Drawing for the job (mm, zero at the part's lowest x, y, z). Give positions to 0.01 mm unless a question says otherwise; leave off trailing zeros. Write each loop counter-clockwise with the first axis right and the second up, starting at its lowest first coordinate (ties: lowest second). Pieces come first, ordered by that corner, then holes. Notation, with made-up numbers: M -3.5,19 L 44.5,19 A13 ccw 44.5,42 Z; hole C -22.75,14 d6. An arc over 180 degrees is marked long. Answer as a JSON object with one key per item and string values. Group by question number.
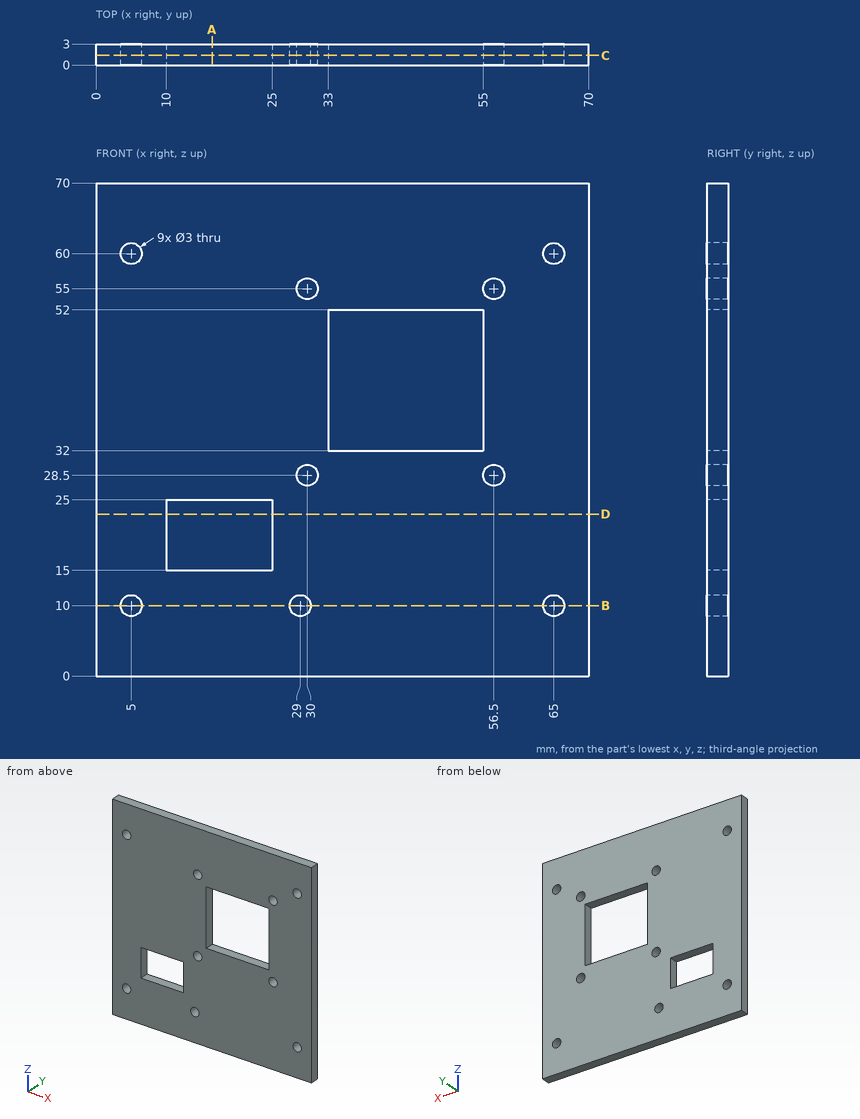
Q1. Slice it at C-C, the plane y = 1.4. Count the separate pieces of the cut face and the enclosed holes in it, then the cut area to 3 significant figures.
Q2. Wall check: L1, parallel to X at y = 1.55, z = 10; L2, parallel to X at y = 1.85, z = 60; L3, parallel to Z at x = 37.5, y = 2. Give the ranges that are in metal, low to high.
Q3. Slice it at A-A, the plane x = 16.5. Write the cut outline in (y, z), then the cut area to 3 significant figures.
Q4. Slice it at D-D, the plane z = 23. Write the cut outline in (x, y), then the cut area to 3 significant figures.
Q5. Drop flat-ended pins along their axis: P1, Ø4, axis at x = 30, z = 55, coming from the +Y side; P2, Ø2.5, axis at x = 65, z = 60, coming from the +Y side. Give the stop position or say it passes through.
Q6. Slice it at B-B, the plane z = 10. Write the cut outline in (x, y).
Solved:
{
 "1": {"separate pieces": "1", "enclosed holes": "11", "area": "4,250 mm²"},
 "2": {"L1": "x = 0 to 3.5, 6.5 to 27.5, 30.5 to 63.5, 66.5 to 70", "L2": "x = 0 to 3.5, 6.5 to 63.5, 66.5 to 70", "L3": "z = 0 to 32, 52 to 70"},
 "3": {"outline": "M 0,0 L 3,0 L 3,15 L 0,15 Z; M 0,25 L 3,25 L 3,70 L 0,70 Z", "area": "180 mm²"},
 "4": {"outline": "M 0,0 L 10,0 L 10,3 L 0,3 Z; M 25,0 L 70,0 L 70,3 L 25,3 Z", "area": "165 mm²"},
 "5": {"P1": "stops at y = 3", "P2": "passes through"},
 "6": {"outline": "M 0,0 L 3.5,0 L 3.5,3 L 0,3 Z; M 6.5,0 L 27.5,0 L 27.5,3 L 6.5,3 Z; M 30.5,0 L 63.5,0 L 63.5,3 L 30.5,3 Z; M 66.5,0 L 70,0 L 70,3 L 66.5,3 Z"}
}
